```python
from build123d import *

# Parameters (mm, degrees)
CROQUIS1_W              = 5
CROQUIS1_H              = 5
SALIENTE_EXTRUIR1_DEPTH = 16.25
CROQUIS2_R              = 2
CORTAR_EXTRUIR1_DEPTH   = 18.184658856


with BuildPart() as part:
    # Croquis1 → Saliente-Extruir1 (new, symmetric)
    with BuildSketch(Plane(origin=(0, 0, 0), x_dir=(1, 0, 0), z_dir=(0, 1, 0))):
        Rectangle(CROQUIS1_W, CROQUIS1_H)
    extrude(amount=SALIENTE_EXTRUIR1_DEPTH, both=True)

    # Croquis2 → Cortar-Extruir1 (cut, through all)
    with BuildSketch(Plane.XY.offset(2.5)):
        with Locations((2.5, 5.25)):
            Circle(CROQUIS2_R)
    extrude(amount=-CORTAR_EXTRUIR1_DEPTH, mode=Mode.SUBTRACT)


solid = part.part
```
Verification items for the finished model (mm, model axes). Round coordinates to 2 decimals unless told otherwise and drop trailing zeros. Order: outer loops, then holes, each group sorted by start corner. A loop starts at its lowest first (then second) coordinate and runs counter-clockwise, first axis right, second up.
1) Depth check by flat-ended pin: pin 1 (1.5 mm diameter, centred on y = 6, z = 0, fed in from +X). Enter the tip coordinate at first touch or a pass-through.
Geometry says:
pin 1: stops at x = 1.18
2) Cross-section at A-A, the plane x = 1.05. Record the cut outline in (y, z).
Geometry says:
outline: (-16.25, -2.5) - (3.87, -2.5) - (3.87, 2.5) - (-16.25, 2.5) - close; (6.63, -2.5) - (16.25, -2.5) - (16.25, 2.5) - (6.63, 2.5) - close
3) Draft check along Y on faces 1 (the flat face through (0, 16.25, 0)), 2 (the cylindrical face through (0.5, 5.3, 0)), 3 (the flat face through (0, -16.25, 0)), 4 (the flat face through (0, 0, 2.5)). Enter one of: +Y half, -Y half, draft (parallel to the pull), parting line (faces both ways), or undercut.
Geometry says:
face 1: +Y half
face 2: undercut
face 3: -Y half
face 4: draft
4) Cross-section at B-B, the plane z = -1.75. Record the cut outline in (x, y).
Geometry says:
outline: (-2.5, -16.25) - (2.5, -16.25) - (2.5, 3.25) arc R2 cw to (2.5, 7.25) - (2.5, 16.25) - (-2.5, 16.25) - close
5) Material ranges on line 1 (Y direction, x = 1.2, z = -1.4); line 2 (Y direction, x = 1.4, z = 0.5); line 3 (X direction, y = 5.5, z = 1.45), recorded low to high.
Geometry says:
line 1: y = -16.25 to 3.73, 6.77 to 16.25
line 2: y = -16.25 to 3.58, 6.92 to 16.25
line 3: x = -2.5 to 0.52
6) Cross-section at C-C, the plane y = 5.25. Record the cut outline in (x, z), plus the area to 3 significant figures.
Geometry says:
outline: (-2.5, -2.5) - (0.5, -2.5) - (0.5, 2.5) - (-2.5, 2.5) - close
area: 15.0 mm2
